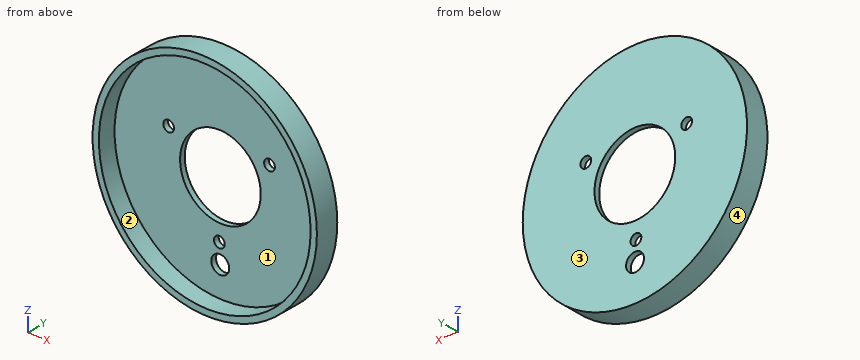
from build123d import *

# Parameters (mm, degrees)
F0_R           = 62.5
F1_DEPTH       = 13
F3_D           = 6
F4_D           = 45
F4_CBORE_D     = 118
F4_CBORE_DEPTH = 10
F5_D           = 10


with BuildPart() as f1:
    # F0 (on Front) → F1 (new body)
    with BuildSketch(Plane.XZ):
        Circle(F0_R)
    extrude(amount=F1_DEPTH)

    # F3 (through all)
    with Locations(Plane.XZ.offset(13)):
        with Locations((-28.862715, 13.725307), (27.342759, 15.962977), (-0.599952, -31.700085)):
            Hole(F3_D / 2)

    # F4 (through all)
    with Locations(Plane.XZ.offset(13)):
        with Locations((4.8e-05, -8.5e-05)):
            CounterBoreHole(F4_D / 2, F4_CBORE_D / 2, F4_CBORE_DEPTH)

    # F5 (through all)
    with Locations(Plane.XZ.offset(13)):
        with Locations((-0.099952, -42.400085)):
            Hole(F5_D / 2)


solid = f1.part
The model under review builds one solid part; all positions refer to its coordinate system, in mm. Face numbers are marked on the shaded views. Give positions to 0.01 mm unless a question says otherwise; leave off trailing zeros. Write each loop counter-clockwise with the first axis right and the second up, starting at its lowest first coordinate (ties: lowest second). Pieces come first, ordered by that corner, then holes. Notation, with made-up numbers: M 16,21.5 L 53,21.5 A11 cw 53,33.5 Z; hole C 38.5,43 d2. An arc over 180 degrees is marked long. One line per question, with ' | ' between items. Start each with the question number.
Item 1: We need section D-D on y = -5.75. Write out the cut boundary in (x, z).
Item 2: We need section A-A on z = 1.5. Write out the cut boundary in (x, y), plus the area to 3 significant figures.
Item 3: Draft analysis for pull direction X (two halves, no side actions). For the marked faces 1, 2, 3 and 4, state which applies: released by +X, released by -X, zero draft, split by the parting line, or undercut.
Item 4: Wall thickness on line 1 (X direction, y = -1.25, z = 14.5); line 2 (X direction, y = -3.5, z = 1); line 3 (Y direction, x = 35.5, z = 28): over which ranges is each line inside the solid? List them lowest first. Write a range as from..to.
Item 5: For pin 1 (4 mm diameter, centred on x = 9, y = -7.5, fed in from +Z); pin 2 (5 mm diameter, centred on x = 26.5, z = -16.5, fed in from -Y); pin 3 (2 mm diameter, centred on y = -8, z = 22, fed in from -X); pin 4 (8 mm diameter, centred on x = -28.86, z = 13.73, fed in from +Y), all flat-tipped, find the tip position at first contact; note any pin that passes through.
Item 6: We need section B-B on x = -20. Write out the cut boundary in (y, z).
Item 7: We need section C-C on x = 0. Write out the cut boundary in (y, z), plus the area to 3 significant figures.
Results found:
1) outline: C 0,0 d125; hole C 0,0 d118
2) outline: M -62.48,-13 L -58.98,-13 L -58.98,-3 L -22.45,-3 L -22.45,0 L -62.48,0 Z; M 22.45,-3 L 58.98,-3 L 58.98,-13 L 62.48,-13 L 62.48,0 L 22.45,0 Z | area: 310 mm2
3) face 1: undercut | face 2: undercut | face 3: zero draft | face 4: split by the parting line
4) line 1: x = -60.79..-31.76, -25.96..-17.2, 17.2..24.72, 29.96..60.79 | line 2: x = -62.49..-58.99, 58.99..62.49 | line 3: y = -3..0
5) pin 1: stops at z = 62.11 | pin 2: stops at y = -3 | pin 3: stops at x = -58.87 | pin 4: stops at y = 0
6) outline: M -13,-59.21 L 0,-59.21 L 0,-10.31 L -3,-10.31 L -3,-55.51 L -13,-55.51 Z; M -13,55.51 L -3,55.51 L -3,10.31 L 0,10.31 L 0,59.21 L -13,59.21 Z
7) outline: M -13,-62.5 L 0,-62.5 L 0,-47.4 L -3,-47.4 L -3,-59 L -13,-59 Z; M -13,59 L -3,59 L -3,22.5 L 0,22.5 L 0,62.5 L -13,62.5 Z; M -3,-37.4 L 0,-37.4 L 0,-34.64 L -3,-34.64 Z; M -3,-28.76 L 0,-28.76 L 0,-22.5 L -3,-22.5 Z | area: 262 mm2
